```python
from build123d import *

# Parameters (mm, degrees)
CYLINDER005_R     = 1.7
CYLINDER005_DEPTH = 30
CYLINDER003_R     = 1.7
CYLINDER003_DEPTH = 30
CYLINDER001_R     = 1.7
CYLINDER001_DEPTH = 30
BOX014_W          = 46.4
BOX014_H          = 8
BOX014_DEPTH      = 2


with BuildPart() as cylinder005:
    # Cylinder005 → Cylinder005 (new body)
    with BuildSketch(Plane(origin=(139, 6.8, -127), x_dir=(1, 0, 0), z_dir=(0, 0, 1))):
        Circle(CYLINDER005_R)
    extrude(amount=CYLINDER005_DEPTH)


with BuildPart() as cylinder003:
    # Cylinder003 → Cylinder003 (new body)
    with BuildSketch(Plane(origin=(118, 6.8, -127), x_dir=(1, 0, 0), z_dir=(0, 0, 1))):
        Circle(CYLINDER003_R)
    extrude(amount=CYLINDER003_DEPTH)


with BuildPart() as cylinder001:
    # Cylinder001 → Cylinder001 (new body)
    with BuildSketch(Plane(origin=(101, 6.8, -127), x_dir=(1, 0, 0), z_dir=(0, 0, 1))):
        Circle(CYLINDER001_R)
    extrude(amount=CYLINDER001_DEPTH)


with BuildPart() as cut008:
    # Box014 → Box014 (new body)
    with BuildSketch(Plane(origin=(96.8, 2.8, -110), x_dir=(1, 0, 0), z_dir=(0, 0, 1))):
        with Locations((23.2, 4)):
            Rectangle(BOX014_W, BOX014_H)
    extrude(amount=BOX014_DEPTH)

    # Cut006: cut Cylinder001
    add(cylinder001.part, mode=Mode.SUBTRACT)

    # Cut007: cut Cylinder003
    add(cylinder003.part, mode=Mode.SUBTRACT)

    # Cut008: cut Cylinder005
    add(cylinder005.part, mode=Mode.SUBTRACT)


solid = cut008.part
```
Model file for the job. Use its own axes, mm. Round coordinates to 2 decimals unless told otherwise and drop trailing zeros. Order: outer loops, then holes, each group sorted by start corner. A loop starts at its lowest first (then second) coordinate and runs counter-clockwise, first axis right, second up. Notation, with made-up numbers: (57, 42) -> (63, 42) arc R15 cw to (63, 57) -> close; hole circle Ø3 at (84.25, -6.5). An arc over 180 degrees is marked (long way). Use one line per item in the form item = value.
Item 1: Pull direction X, two halves, no side cores. Call faces 1 (the face through (140.62, 7.31, -109.01)), 2 (the face through (120, 6, -108)), 3 (the face through (99.3, 6.87, -109.01)), 4 (the face through (143.2, 7, -109)): released by +X, released by -X, zero draft, split by the parting line, or undercut.
Returned:
face_1 = undercut
face_2 = zero draft
face_3 = undercut
face_4 = released by +X
Item 2: Cut at D-D, the plane y = 7.75. Write the cut outline in (x, z).
Returned:
outline = (96.8, -110) -> (99.59, -110) -> (99.59, -108) -> (96.8, -108) -> close; (102.41, -110) -> (116.59, -110) -> (116.59, -108) -> (102.41, -108) -> close; (119.41, -110) -> (137.59, -110) -> (137.59, -108) -> (119.41, -108) -> close; (140.41, -110) -> (143.2, -110) -> (143.2, -108) -> (140.41, -108) -> close
Item 3: Drill centre lines: line 1 (X direction, y = 6.8, z = -108.45); line 2 (Y direction, x = 118, z = -108.75); line 3 (Y direction, x = 119, z = -108.15). Where is each one in solid material? Low to high.
Returned:
line_1 = 96.8 to 99.3, 102.7 to 116.3, 119.7 to 137.3, 140.7 to 143.2
line_2 = 2.8 to 5.1, 8.5 to 10.8
line_3 = 2.8 to 5.43, 8.17 to 10.8
Item 4: Cut at C-C, the plane z = -108.9. Write the cut outline in (x, y), and give its area (3 significant figures).
Returned:
outline = (96.8, 2.8) -> (143.2, 2.8) -> (143.2, 10.8) -> (96.8, 10.8) -> close; hole circle Ø3.4 at (101, 6.8); hole circle Ø3.4 at (118, 6.8); hole circle Ø3.4 at (139, 6.8)
area = 344 mm^2
Item 5: Cut at A-A, the plane y = 6. Write the cut outline in (x, z).
Returned:
outline = (96.8, -110) -> (99.5, -110) -> (99.5, -108) -> (96.8, -108) -> close; (102.5, -110) -> (116.5, -110) -> (116.5, -108) -> (102.5, -108) -> close; (119.5, -110) -> (137.5, -110) -> (137.5, -108) -> (119.5, -108) -> close; (140.5, -110) -> (143.2, -110) -> (143.2, -108) -> (140.5, -108) -> close
Item 6: Cut at B-B, the plane x = 118. Write the cut outline in (y, z), and give its area (3 significant figures).
Returned:
outline = (2.8, -110) -> (5.1, -110) -> (5.1, -108) -> (2.8, -108) -> close; (8.5, -110) -> (10.8, -110) -> (10.8, -108) -> (8.5, -108) -> close
area = 9.20 mm^2
